Verification items for the finished model (mm, model axes). Round coordinates to 2 decimals unless told otherwise and drop trailing zeros. Loops run counter-clockwise (first coordinate to the right, second up) from the corner with the lowest first, then second, coordinate; pieces in that order, holes last. Notation, with made-up numbers: M -2,12.25 L 51,12.25 A33 ccw 51,42.25 Z; hole C 81.5,57.25 d8. An arc over 180 degrees is marked long. Answer as CSV lines item,"result".
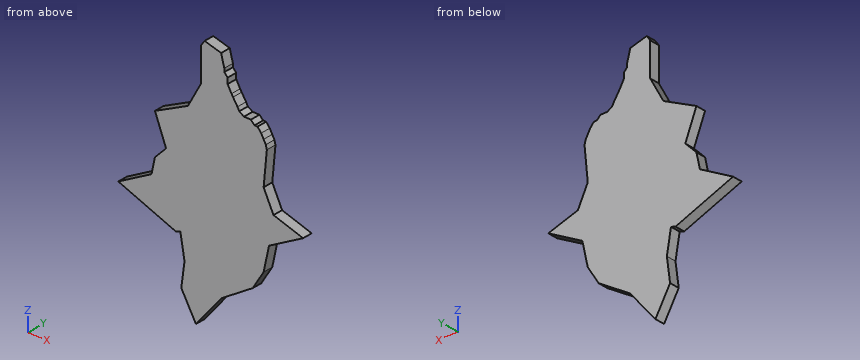
```python
from build123d import *

# Parameters (mm, degrees)
F1_DEPTH = 3
F2_SCALE = 0.6


with BuildPart() as f1:
    # F0 (on Front) → F1 (new body)
    with BuildSketch(Plane.XZ):
        Polygon((1.3910490088, 38.3051857352), (-3.6360053346, 39.6043136716), (-4.6649789438, 38.0779765546), (-4.6649789438, 28.0484538525), (-8.694652468, 20.5713305622), (-18.7318380922, 15.4852615669), (-15.3588512912, 6.848028861), (-18.7413649335, 3.2623104389), (-19.7978429212, -1.5990479397), (-29.8871286213, -7.3253973387), (-12.3931569979, -13.9208259061), (-11.0025182366, -13.4662510827), (-9.7458269447, -20.7670312375), (-10.7237989575, -28.1813337487), (-6.2755574472, -36.0187143087), (1.4870599844, -26.3149570674), (10.9971901402, -20.069969818), (14.3194012509, -14.5789282396), (15.9598111512, -7.0306210286), (26.3209752738, -1.149962307), (17.3118170351, 1.5612578718), (14.3194012509, 7.7631301247), (15.2990790084, 18.0060230196), (14.9825164439, 19.2469840983), (14.3194012509, 20.4153303112), (13.5617544875, 21.7502322048), (12.4618653208, 23.0545718223), (11.5581247956, 23.0545718223), (10.428449139, 24.1277627647), (8.3385501057, 24.1277627647), (6.9153775882, 25.0160566247), (6.3616191037, 25.9917266667), (5.0060097128, 28.0251428485), (4.5541389845, 28.7594310939), (3.3679804765, 30.8493301272), (3.3679804765, 32.5438417494), (2.3512728512, 33.6170345545), (2.3512728512, 34.6337407827), align=None)
    extrude(amount=F1_DEPTH)


with BuildPart() as f1_1:
    # F2: moved
    add(f1.part.scale(F2_SCALE).moved(Location((-2.5102229789, -1.2, -14.4074857235))))


solid = f1_1.part
```
1) Section check A-A (z = -14). Record the cut outline in (x, y).
Here are the results:
outline,"M -14.09,-3 L 9.64,-3 L 9.64,-1.2 L -14.09,-1.2 Z"
2) Go/stop test with flat-tipped pins: pin 1 (1.5 mm diameter, centred on x = 6.5, z = -21.5, fed in from -Y); pin 2 (0.6 mm diameter, centred on x = 5, y = -2, fed in from +Z); pin 3 (0.5 mm diameter, centred on y = -2, z = 5, fed in from +X); pin 4 (0.6 mm diameter, centred on x = 3.5, y = -2, fed in from +Z). Record where each tip stops, or that it passes through.
Here are the results:
pin 1,"stops at y = -3"
pin 2,"stops at z = -0.57"
pin 3,"stops at x = -0.49"
pin 4,"stops at z = 0.07"
3) Section check B-B (x = -3). Record the cut outline in (y, z), plus the area to 3 significant figures.
Here are the results:
outline,"M -3,-31.92 L -1.2,-31.92 L -1.2,8.92 L -3,8.92 Z"
area,"73.5 mm^2"
4) Material ranges on probe 1 along X at (y, z) = (-2.6, 6); probe 2 along Z at (x, y) = (-19, -2.45); probe 3 along Z at (x, y) = (-16.5, -1.95), recorded low to high.
Here are the results:
probe 1,"x = -5.31 to -1.1"
probe 2,"z = -19.35 to -17.98"
probe 3,"z = -20.29 to -16.57"
